Part print with two shaded views. Sizes in mm from the minimum x, y, z corner. A direction names the side the tool comes from. Give positions to 0.01 mm unless a question says otherwise; leave off trailing zeros. Order: outer loops, then holes, each group sorted by start corner. A loop starts at its lowest first (then second) coordinate and runs counter-clockwise, first axis right, second up. Notation, with made-up numbers: M 77.5,46 L 120.5,46 A23 ccw 120.5,66 Z; hole C -31,-28 d8. An arc over 180 degrees is marked long. Write each question's results on one line, items separated by ' | '. Start each with the question number.
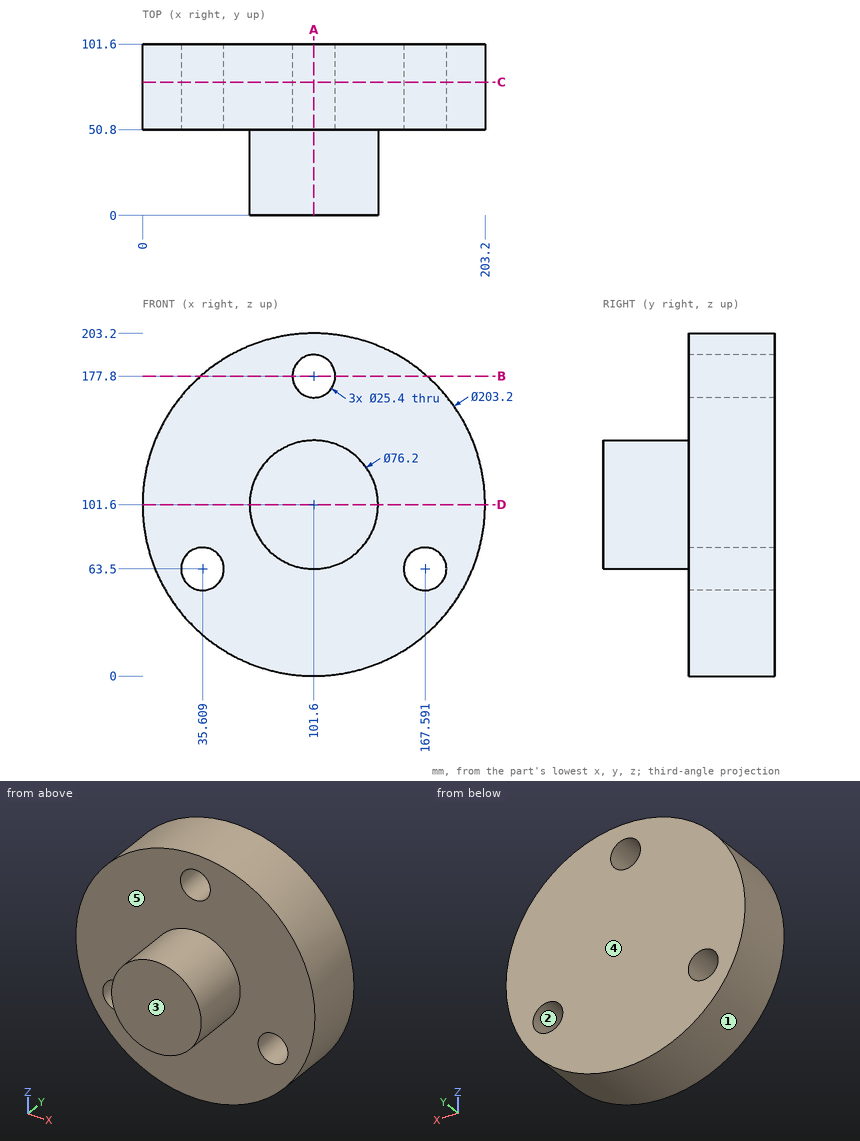
(1) Saw through at B-B on z = 177.8. Give the cut face in (x, y), plus the area to 3 significant figures.
(2) Probe L1, parallel to Z at x = 101.6, y = 78; L2, parallel to Y at x = 157.5, z = 47.5; L3, parallel to Z at x = 92, y = 61.5 (1 decimal). List the from-to ranges inside material, lowest first.
(3) Drop flat-ended pins along their axis: P1, Ø8, axis at x = 63, y = 31.5, coming from the +Z side; P2, Ø1.5, axis at x = 128, z = 49.5, coming from the -Y side; P3, Ø1.5, axis at x = 49, y = 51.5, coming from the +Z side. Give the stop position or say it passes through.
(4) Pull direction X, two halves, no side cores. Call the marked faces 1, 2 and 3: +X half, -X half, draft (parallel to the pull), parting line (faces both ways), or undercut.
(5) Tool access for the marked faces 4 and 5: list every direction of +Z, -Z, +X, -X, +Y, -Y with a clear straight run to the whole face (end or side of a thin tool).
(6) Saw through at D-D on z = 101.6. Give the cut face in (x, y), plus the area to 3 significant figures.
(7) Saw through at A-A on x = 101.6. Give the cut face in (y, z), plus the area to 3 significant figures.
(8) Saw through at C-C on y = 79. Give the cut face in (x, z).
Taken from the geometry:
1) outline: M 34.4,50.8 L 88.9,50.8 L 88.9,101.6 L 34.4,101.6 Z; M 114.3,50.8 L 168.8,50.8 L 168.8,101.6 L 114.3,101.6 Z | area: 5,540 mm²
2) L1: z = 0 to 165.1, 190.5 to 203.2 | L2: y = 50.8 to 101.6 | L3: z = 0.5 to 169.5, 186.1 to 202.7
3) P1: stops at z = 117.55 | P2: stops at y = 50.8 | P3: stops at z = 188.97
4) face 1: parting line | face 2: undercut | face 3: draft
5) face 4: +Z, -Z, +X, -X, +Y | face 5: -Y
6) outline: M 0,50.8 L 63.5,50.8 L 63.5,0 L 139.7,0 L 139.7,50.8 L 203.2,50.8 L 203.2,101.6 L 0,101.6 Z | area: 14,200 mm²
7) outline: M 0,63.5 L 50.8,63.5 L 50.8,0 L 101.6,0 L 101.6,165.1 L 50.8,165.1 L 50.8,139.7 L 0,139.7 Z; M 50.8,190.5 L 101.6,190.5 L 101.6,203.2 L 50.8,203.2 Z | area: 12,900 mm²
8) outline: C 101.6,101.6 d203.2; hole C 35.61,63.5 d25.4; hole C 101.6,177.8 d25.4; hole C 167.59,63.5 d25.4
